Design review of the part built by this model. Coordinates are the model's own, in mm. Face numbers are marked on the shaded views. A direction names the side the tool comes from. Coordinates: 2 decimals unless noted, no trailing zeros. Write each loop counter-clockwise with the first axis right and the second up, starting at its lowest first coordinate (ties: lowest second). Pieces come first, ordered by that corner, then holes. Notation, with made-up numbers: (-2, 44) - (30, 44) arc R15 ccw to (30, 68) - close; hole circle Ø9 at (-35.75, 37). An arc over 180 degrees is marked (long way). One line per item, written item: value.
Autodesk Inventor part; units mm, degrees
ref_plane "YZ Plane" through (0, 0, 0) normal (1, 0, 0) x (0, 1, 0)
ref_plane "XZ Plane" through (0, 0, 0) normal (0, 1, 0) x (-1, 0, 0)
ref_plane "XY Plane" through (0, 0, 0) normal (0, 0, 1) x (1, 0, 0)
sketch "Sketch1" plane through (0, 0, 0) normal (0, 0, 1) x (1, 0, 0)
  line L0 (-44.577, -50) -> (44.577, -50)
  line L1 (44.577, -50) -> (44.577, 50)
  line L2 (44.577, 50) -> (-44.577, 50)
  line L3 (-44.577, 50) -> (-44.577, -50)
  line L4 (54.577, 60) -> (54.577, -60)
  line L5 (54.577, -60) -> (-54.577, -60)
  line L6 (-54.577, -60) -> (-54.577, 60)
  line L7 (-54.577, 60) -> (54.577, 60)
  circle A0 centre (34.337, -9.9) radius 1.7
  circle A1 centre (34.337, 20.6) radius 1.7
  circle A2 centre (-40.163, -9.9) radius 1.7
  circle A3 centre (-40.163, 20.6) radius 1.7
  point P0 (0, 0)
  dimension "d0" = 10
extrude "Extrusion1" add sketch "Sketch1" along normal blind 5 contours L3 L2 L1 L0 | L4 L5 L6 L7
sketch "Sketch2" plane through (0, 0, 0) normal (0, 0, -1) x (-1, 0, 0)
  line L0 (44.577, -50) -> (-44.577, -50)
  line L1 (44.577, 50) -> (44.577, -50)
  line L2 (-44.577, 50) -> (44.577, 50)
  line L3 (-44.577, -50) -> (-44.577, 50)
  line L4 (54.577, 60) -> (54.577, -60)
  line L5 (-54.577, 60) -> (54.577, 60)
  line L6 (-54.577, -60) -> (-54.577, 60)
  line L7 (54.577, -60) -> (-54.577, -60)
  circle A0 centre (-34.337, -9.9) radius 1.7
  circle A1 centre (-34.337, 20.6) radius 1.7
  circle A2 centre (40.163, -9.9) radius 1.7
  circle A3 centre (40.163, 20.6) radius 1.7
  line L8 (47.077, 52.5) -> (47.077, -52.5)
  line L9 (47.077, -52.5) -> (-47.077, -52.5)
  line L10 (-47.077, -52.5) -> (-47.077, 52.5)
  line L11 (-47.077, 52.5) -> (47.077, 52.5)
  line L12 (52.077, 57.5) -> (52.077, -57.5)
  line L13 (52.077, -57.5) -> (-52.077, -57.5)
  line L14 (-52.077, -57.5) -> (-52.077, 57.5)
  line L15 (-52.077, 57.5) -> (52.077, 57.5)
  point P0 (0, 0)
  dimension "d3" = 2.5
  dimension "d4" = 2.5
extrude "Extrusion2" add sketch "Sketch2" along normal blind 11.75 contours L12 L13 L14 L15
fillet "Fillet1" radius 2 7 edges at (52.077, -57.5, -5.875) (54.577, -60, 2.5) (-54.577, -60, 2.5) (-54.577, 60, 2.5) (-52.077, 57.5, -5.875) (52.077, 57.5, -5.875) (54.577, 60, 2.5)
sketch "Sketch3" plane through (-52.077, -57.5, -11.75) normal (0, -1, 0) x (1, 0, 0)
  line L0 (44.1897, 5.1489) -> (44.1897, 11.75)
  line L1 (60.1104, 5.1489) -> (44.1897, 5.1489)
  line L2 (60.1104, 11.75) -> (60.1104, 5.1489)
  line L3 (0, 11.75) -> (102.154, 11.75)
  point P0 (52.077, 11.75)
extrude "Extrusion3" cut sketch "Sketch3" against normal blind 11.75
sketch "Sketch4" plane through (-50.077, 57.5, 0) normal (0, 1, 0) x (1, 0, 0)
  line L0 (40.077, 10) -> (60.077, 10)
  line L1 (40.077, 0) -> (40.077, 10)
  line L2 (60.077, 10) -> (60.077, 0)
  line L3 (100.154, 0) -> (0, 0)
  point P0 (50.077, 0)
extrude "Extrusion4" cut sketch "Sketch4" against normal blind 11.75
properties part number "Cubierta parte 1"
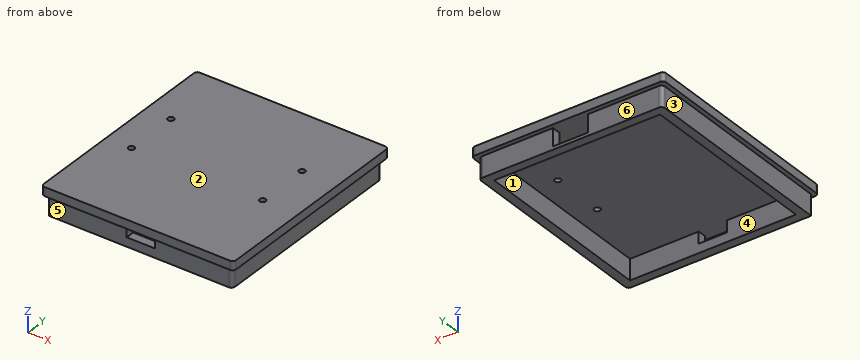
1. Consider section A-A, the plane y = 20.6. Write out the cut boundary in (x, z), then the cut area to 3 significant figures.
Answer block:
outline: (-54.58, 0) - (-52.08, 0) - (-52.08, -11.75) - (-47.08, -11.75) - (-47.08, 0) - (-41.86, 0) - (-41.86, 5) - (-54.58, 5) - close; (-38.46, 0) - (32.64, 0) - (32.64, 5) - (-38.46, 5) - close; (36.04, 0) - (47.08, 0) - (47.08, -11.75) - (52.08, -11.75) - (52.08, 0) - (54.58, 0) - (54.58, 5) - (36.04, 5) - close
area: 629 mm^2
2. Consider section C-C, the plane x = 2. Write out the cut boundary in (y, z), then the cut area to 3 significant figures.
Answer block:
outline: (-60, 0) - (60, 0) - (60, 5) - (-60, 5) - close; (-57.5, -11.75) - (-52.5, -11.75) - (-52.5, -6.6) - (-57.5, -6.6) - close; (52.5, -11.75) - (57.5, -11.75) - (57.5, -10) - (52.5, -10) - close
area: 634 mm^2
3. Consider section B-B, the plane z = -2.25. Write out the cut boundary in (x, y).
Answer block:
outline: (-52.08, -57.5) - (-7.89, -57.5) - (-7.89, -52.5) - (-47.08, -52.5) - (-47.08, 52.5) - (-10, 52.5) - (-10, 57.5) - (-50.08, 57.5) arc R2 ccw to (-52.08, 55.5) - close; (8.03, -57.5) - (50.08, -57.5) arc R2 ccw to (52.08, -55.5) - (52.08, 55.5) arc R2 ccw to (50.08, 57.5) - (10, 57.5) - (10, 52.5) - (47.08, 52.5) - (47.08, -52.5) - (8.03, -52.5) - close
4. Insertion check: pin 1 Ø2.5 at (y, z) = (54, -6.5) entering from +X; pin 2 Ø5 at (x, y) = (17, 30) entering from -Z; pin 3 Ø3 at (x, z) = (-28.5, -2.5) entering from +Y. Each pin has a flat end and moves straight along its axis. Give the tip position at first contact, or say it passes through.
Answer block:
pin 1: stops at x = 52.08
pin 2: stops at z = 0
pin 3: stops at y = 57.5
5. Wall thickness on line 1 along X through (y, z) = (26, -8); line 2 along Y through (x, z) = (24.5, -5.25); line 3 along Z through (x, y) = (-9, 12): over which ranges is each line inside the solid? List them lowest first.
Answer block:
line 1: x = -52.08 to -47.08, 47.08 to 52.08
line 2: y = -57.5 to -52.5, 52.5 to 57.5
line 3: z = 0 to 5
6. Mouldability with a two-part tool opening along Y and no side actions: class the marked faces 3, 4, 5 and 6 as released by +Y, released by -Y, zero draft, split by the parting line, or undercut.
Answer block:
face 3: zero draft
face 4: undercut
face 5: released by -Y
face 6: released by +Y
7. Consider section D-D, the plane x = 31. Write out the cut boundary in (y, z).
Answer block:
outline: (-60, 0) - (-57.5, 0) - (-57.5, -11.75) - (-52.5, -11.75) - (-52.5, 0) - (52.5, 0) - (52.5, -11.75) - (57.5, -11.75) - (57.5, 0) - (60, 0) - (60, 5) - (-60, 5) - close
8. For the marked faces 1 and 2, list the 3-axis set-ups (+Z, -Z, +X, -X, +Y, -Y) from which the entire face can be reached by the end or side of a thin tool; tool diameter is ignored.
Answer block:
face 1: -Z
face 2: +Z, +X, -X, +Y, -Y
